```python
from build123d import *

# Parameters (mm, degrees)
EXTRUDE_1_DEPTH      = 70
EXTRUDE_3_DEPTH      = 5
EXTRUDE_3_DEPTH_BACK = 10
SKETCH_2_R           = 2.5


with BuildPart() as part:
    # 草图1 → 凸台-拉伸1 (new body)
    with BuildSketch(Plane.XY):
        with BuildLine():
            Line((-28, 9.5), (28, 9.5))
            ThreePointArc((28, 9.5), (37.5, 0), (28, -9.5))
            Line((28, -9.5), (-28, -9.5))
            ThreePointArc((-28, -9.5), (-37.5, 0), (-28, 9.5))
        make_face()
    extrude(amount=EXTRUDE_1_DEPTH)

    # 草图2 → 凸台-拉伸3 (add, two sides: drawn at the far end of the back side and taken through both)
    with BuildSketch(Plane.ZY.offset(37.5).offset(-EXTRUDE_3_DEPTH_BACK)):
        with Locations((2.5, 0)):
            Circle(SKETCH_2_R)
    extrude(amount=EXTRUDE_3_DEPTH + EXTRUDE_3_DEPTH_BACK)


solid = part.part
```
Check sheet for the modelled part. Datum: model origin and axes. Units: mm. A direction names the side the tool comes from. Round coordinates to 2 decimals unless told otherwise and drop trailing zeros. Order: outer loops, then holes, each group sorted by start corner. A loop starts at its lowest first (then second) coordinate and runs counter-clockwise, first axis right, second up. Notation, with made-up numbers: M -2,47.25 L 43,47.25 A21 ccw 43,60.25 Z; hole C 33,73 d11. An arc over 180 degrees is marked long. Answer in a Markdown table with one row per item.
(1) Gauge pin test, flat ends, axial feed: pin 1 (3 mm diameter, centred on y = 3, z = 19, fed in from +X); pin 2 (4 mm diameter, centred on y = 6.5, z = 35, fed in from -X); pin 3 (8 mm diameter, centred on y = -4, z = 42.5, fed in from -X). Record the tip position at first contact, or that the pin passes through.
Findings:
| item | result |
|---|---|
| pin 1 | stops at x = 37.38 |
| pin 2 | stops at x = -36.37 |
| pin 3 | stops at x = -37.5 |
(2) Section check D-D on z = 59.5. Record the boundary of the cut face in (x, y).
Findings:
| item | result |
|---|---|
| outline | M -28,-9.5 L 28,-9.5 A9.5 ccw 28,9.5 L -28,9.5 A9.5 ccw Z |
(3) Set-up check for faces 1 (the flat face through (1, 0, 0)), 2 (the cylindrical face through (-40, 0, 0)): record each of +Z, -Z, +X, -X, +Y, -Y from which the full face is reachable in a straight line by a thin tool's end or side.
Findings:
| item | result |
|---|---|
| face 1 | -Z, +X, -X, +Y, -Y |
| face 2 | -X |
(4) Section check B-B on y = -1. Record the boundary of the cut face in (x, z), plus the area to 3 significant figures.
Findings:
| item | result |
|---|---|
| outline | M -42.5,0.21 L -37.45,0.21 L -37.45,0 L 37.45,0 L 37.45,70 L -37.45,70 L -37.45,4.79 L -42.5,4.79 Z |
| area | 5,270 mm^2 |
(5) Material ranges on line 1 along X through (y, z) = (0.5, 49); line 2 along X through (y, z) = (3.5, 65); line 3 along Y through (x, z) = (-30, 34), recorded low to high. Write a range as from..to.
Findings:
| item | result |
|---|---|
| line 1 | x = -37.49..37.49 |
| line 2 | x = -36.83..36.83 |
| line 3 | y = -9.29..9.29 |
(6) Section check A-A on z = 2.5. Record the boundary of the cut face in (x, y), plus the area to 3 significant figures.
Findings:
| item | result |
|---|---|
| outline | M -42.5,-2.5 L -37.17,-2.5 A9.5 ccw -28,-9.5 L 28,-9.5 A9.5 ccw 28,9.5 L -28,9.5 A9.5 ccw -37.17,2.5 L -42.5,2.5 Z |
| area | 1,370 mm^2 |
(7) Section check C-C on y = -5. Record the boundary of the cut face in (x, z), plus the area to 3 significant figures.
Findings:
| item | result |
|---|---|
| outline | M -36.08,0 L 36.08,0 L 36.08,70 L -36.08,70 Z |
| area | 5,050 mm^2 |
